from build123d import *

# Parameters (mm, degrees)
PAD_DEPTH       = 40
SKETCH001_R     = 16
POCKET_DEPTH    = 35
POCKET001_DEPTH = 4
SKETCH003_R     = 2.6
POCKET002_DEPTH = 30
CHAMFER_SIZE    = 6


with BuildPart() as part:
    # Sketch → Pad (new body)
    with BuildSketch(Plane.XY):
        with BuildLine():
            Line((-50, 40), (6.755886, 24.069857))
            ThreePointArc((6.755886, -24.069857), (25, 0), (6.755886, 24.069857))
            Line((6.755886, -24.069857), (-50, -40))
            Line((-50, 40), (-50, -40))
        make_face()
    extrude(amount=PAD_DEPTH)

    # Sketch001 (on Face6 of Pad) → Pocket (cut)
    with BuildSketch(Plane.XY.offset(40)):
        Circle(SKETCH001_R)
    extrude(amount=-POCKET_DEPTH, mode=Mode.SUBTRACT)

    # Sketch002 (on Face2 of Pocket) → Pocket001 (cut)
    with BuildSketch(Plane(origin=(-44, 0, 0), x_dir=(0, -1, 0), z_dir=(-1, 0, 0))):
        Polygon((-29.05, 31.661731), (-25, 29.323463), (-20.95, 31.661731), (-20.95, 51.661731), (-29.05, 51.661731), align=None)
        Polygon((25, 29.323463), (20.95, 31.661731), (20.95, 51.661731), (29.05, 51.661731), (29.05, 31.661731), align=None)
        Polygon((-29.05, 8.338269), (-25, 10.676537), (-20.95, 8.338269), (-20.95, -11.661731), (-29.05, -11.661731), align=None)
        Polygon((20.95, 8.338269), (25, 10.676537), (29.05, 8.338269), (29.05, -11.661731), (20.95, -11.661731), align=None)
    extrude(amount=-POCKET001_DEPTH, mode=Mode.SUBTRACT)

    # Sketch003 (on Face2 of Pocket001) → Pocket002 (cut)
    with BuildSketch(Plane(origin=(-50, 0, 0), x_dir=(0, -1, 0), z_dir=(-1, 0, 0))):
        with Locations((25, 34)):
            Circle(SKETCH003_R)
        with Locations((-25, 6)):
            Circle(SKETCH003_R)
        with Locations((25, 6)):
            Circle(SKETCH003_R)
        with Locations((-25, 34)):
            Circle(SKETCH003_R)
    extrude(amount=-POCKET002_DEPTH, mode=Mode.SUBTRACT)

    # Chamfer
    chamfer_edges = [part.edges().sort_by_distance(p)[0] for p in [
        (-21.622057, -32.034928, 40),
        (-21.622057, -32.034928, 0),
    ]]
    chamfer(chamfer_edges, length=CHAMFER_SIZE)


solid = part.part
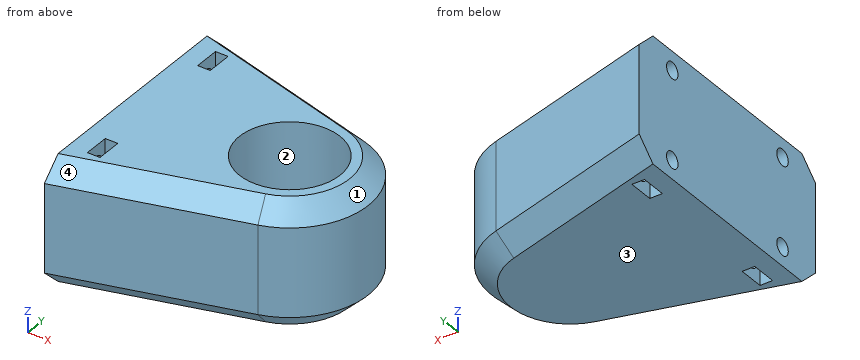
Work out the finished part from the listing and answer in its coordinate system (mm). Face numbers are marked on the shaded views. Coordinates: 2 decimals unless noted, no trailing zeros. Write each loop counter-clockwise with the first axis right and the second up, starting at its lowest first coordinate (ties: lowest second). Pieces come first, ordered by that corner, then holes.
1. Flat-ended cylindrical pins translate along their axes: pin 1 (12 mm diameter, centred on x = -23, z = 4.5, fed in from -Y); pin 2 (1.2 mm diameter, centred on x = -42, z = 3.5, fed in from -Y); pin 3 (3 mm diameter, centred on x = -41.5, z = 4, fed in from +Y); pin 4 (9 mm diameter, centred on y = -23.5, z = 35.5, fed in from -X). Find the tip coordinate at first contact, or state that the pin passes through.
Results list:
pin 1: stops at y = -34.05
pin 2: stops at y = -35.8
pin 3: stops at y = 37.15
pin 4: stops at x = -50
2. Consider line 1 along Z through (x, y) = (-24, -25); line 2 along Z through (x, y) = (-1, -10.5); line 3 along X through (y, z) = (-1, 37). Determine where each line is inside the solid, lowest interval first.
Results list:
line 1: z = 0 to 3.4, 8.6 to 31.4, 36.6 to 40
line 2: z = 0 to 5
line 3: x = -50 to -15.97, 15.97 to 21.98
3. For a pull along Y with two mould halves and no side action, classify the marked faces 1, 2, 3 and 4 as +Y half, -Y half, draft (parallel to the pull), parting line (faces both ways), or undercut.
Results list:
face 1: parting line
face 2: undercut
face 3: draft
face 4: -Y half
4. The part is cut by section D-D, the plane y = 26. State how many separate pieces and enclosed holes the cut face has, and give its area (3 significant figures).
Results list:
separate pieces: 3
enclosed holes: 0
area: 1,530 mm2
5. The part is cut by section A-A, the plane z = 21.5. Write down the section's boundary in (x, y), and give its area (3 significant figures).
Results list:
outline: (-50, -40) - (6.76, -24.07) arc R25 ccw to (6.76, 24.07) - (-50, 40) - close; hole circle Ø32 at (0, 0)
area: 3,480 mm2
6. The part is cut by section B-B, the plane x = -30. Write down the section's boundary in (y, z).
Results list:
outline: (-34.39, 6) - (-28.15, 0) - (28.15, 0) - (34.39, 6) - (34.39, 34) - (28.15, 40) - (-28.15, 40) - (-34.39, 34) - close; hole circle Ø5.2 at (-25, 6); hole circle Ø5.2 at (-25, 34); hole circle Ø5.2 at (25, 6); hole circle Ø5.2 at (25, 34)
7. The part is cut by section C-C, the plane y = 0. Write down the section's boundary in (x, z).
Results list:
outline: (-50, 0) - (19, 0) - (25, 6) - (25, 34) - (19, 40) - (16, 40) - (16, 5) - (-16, 5) - (-16, 40) - (-50, 40) - close
